```python
from build123d import *

# Parameters (mm, degrees)
SKETCH1_R           = 7.5
BOSS_EXTRUDE1_DEPTH = 16
SKETCH2_R           = 8.5
BOSS_EXTRUDE2_DEPTH = 2
SKETCH3_R           = 7
BOSS_EXTRUDE3_DEPTH = 35
SKETCH4_R           = 4
CUT_EXTRUDE1_DEPTH  = 20.5
SKETCH6_W           = 3
SKETCH6_H           = 1.5
CUT_EXTRUDE2_DEPTH  = 20.5
CUT_EXTRUDE3_REACH  = 18
SKETCH7_R           = 1
SKETCH8_W           = 3
SKETCH8_H           = 3
CUT_EXTRUDE5_DEPTH  = 33


with BuildPart() as part:
    # Sketch1 → Boss-Extrude1 (new body)
    with BuildSketch(Plane(origin=(0, 0, 0), x_dir=(0, 0, -1), z_dir=(1, 0, 0))):
        Circle(SKETCH1_R)
    extrude(amount=BOSS_EXTRUDE1_DEPTH)

    # Sketch2 → Boss-Extrude2 (add)
    with BuildSketch(Plane(origin=(16, 0, 0), x_dir=(0, 0, -1), z_dir=(1, 0, 0))):
        Circle(SKETCH2_R)
    extrude(amount=BOSS_EXTRUDE2_DEPTH)

    # Sketch3 → Boss-Extrude3 (add)
    with BuildSketch(Plane(origin=(18, 0, 0), x_dir=(0, 0, -1), z_dir=(1, 0, 0))):
        Circle(SKETCH3_R)
    extrude(amount=BOSS_EXTRUDE3_DEPTH)

    # Sketch4 → Cut-Extrude1 (cut)
    with BuildSketch(Plane.ZY):
        Circle(SKETCH4_R)
    extrude(amount=-CUT_EXTRUDE1_DEPTH, mode=Mode.SUBTRACT)

    # Sketch6 → Cut-Extrude2 (cut)
    with BuildSketch(Plane.ZY):
        with Locations((0, 4)):
            Rectangle(SKETCH6_W, SKETCH6_H)
    extrude(amount=-CUT_EXTRUDE2_DEPTH, mode=Mode.SUBTRACT)

    # Sketch7 → Cut-Extrude3 (cut, up to next)
    with BuildSketch(Plane(origin=(0, 7.5, 0), x_dir=(1, 0, 0), z_dir=(0, 1, 0)), mode=Mode.PRIVATE) as cut_extrude3_sk1:
        with Locations((9.6, 0)):
            Circle(SKETCH7_R)
    cut_extrude3_tool1 = extrude(cut_extrude3_sk1.sketch, amount=-CUT_EXTRUDE3_REACH, mode=Mode.PRIVATE) & part.part
    add(cut_extrude3_tool1.solids().sort_by_distance((9.6, 7.5, 0))[0], mode=Mode.SUBTRACT)

    # Sketch8 → Cut-Extrude5 (cut)
    with BuildSketch(Plane(origin=(53, 0, 0), x_dir=(0, 0, -1), z_dir=(1, 0, 0))):
        with Locations((0, -7)):
            Rectangle(SKETCH8_W, SKETCH8_H)
    extrude(amount=-CUT_EXTRUDE5_DEPTH, mode=Mode.SUBTRACT)


solid = part.part
```
CAD build for the part. Positions are in the model's coordinates, mm. A direction names the side the tool comes from. Give positions to 0.01 mm unless a question says otherwise; leave off trailing zeros. Write each loop counter-clockwise with the first axis right and the second up, starting at its lowest first coordinate (ties: lowest second). Pieces come first, ordered by that corner, then holes. Notation, with made-up numbers: (12, -11.5) -> (19, -11.5) arc R20 ccw to (19, 23.5) -> close; hole circle Ø6 at (56, 31). An arc over 180 degrees is marked (long way). Write each question's results on one line, items separated by ' | '.
1. Cut at C-C, the plane x = 12. Write the cut outline in (y, z).
Geometry check:
outline: circle Ø15 at (0, 0); hole (3.71, -1.5) -> (4.75, -1.5) -> (4.75, 1.5) -> (3.71, 1.5) arc R4 ccw (long way) to start
2. Drop flat-ended pins along their axis: P1, Ø0.7, axis at x = 39, y = -6, coming from the -Z side; P2, Ø6.5, axis at y = -1, z = -1, coming from the -X side; P3, Ø4, axis at x = 6.5, y = -2, coming from the -Z side; P4, Ø4, axis at x = 25, y = 4, coming from the -Z side. Give the stop position or say it passes through.
Geometry check:
P1: z = -4.13 | P2: x = 0 | P3: z = -7.5 | P4: z = -6.71
3. Cut at A-A, the plane z = 0. Write the cut outline in (x, y), then the cut area to 3 significant figures.
Geometry check:
outline: (0, -7.5) -> (16, -7.5) -> (16, -8.5) -> (18, -8.5) -> (18, -7) -> (20, -7) -> (20, -5.5) -> (53, -5.5) -> (53, 7) -> (18, 7) -> (18, 8.5) -> (16, 8.5) -> (16, 7.5) -> (10.6, 7.5) -> (10.6, 4.75) -> (20.5, 4.75) -> (20.5, -4) -> (0, -4) -> close; (0, 4.75) -> (8.6, 4.75) -> (8.6, 7.5) -> (0, 7.5) -> close | area: 530 mm²
4. Which spindle directions (+Z, -Z, +X, -X, +Y, -Y) get a long thin tool onto all of the face, cutting with end or side? Do faces 1 (the flat face through (53, 0, 0)), 2 (the flat face through (37, -6, 1.5)), 3 (the cylindrical face through (10.524, 6.144, 0.383)), 4 (the cylindrical face through (35.255, -2.681, -6.466)), 5 (the flat face through (16, -8, 0)). Say none if no direction does.
Geometry check:
face 1: +Z, -Z, +X, +Y, -Y | face 2: +X, -Y | face 3: +Y | face 4: +X | face 5: -X
5. Wall check: probe 1 along Y at (x, z) = (5.25, 0); probe 2 along Y at (x, z) = (19.5, 0.25); probe 3 along X at (y, z) = (-2, -0.25). Give the ranges that are in metal, low to high. Write a range as [from, to].
Geometry check:
probe 1: [-7.5, -4], [4.75, 7.5] | probe 2: [-7, -3.99], [4.75, 7] | probe 3: [20.5, 53]
6. Cut at B-B, the plane y = 0. Write the cut outline in (x, z).
Geometry check:
outline: (0, -7.5) -> (16, -7.5) -> (16, -8.5) -> (18, -8.5) -> (18, -7) -> (53, -7) -> (53, 7) -> (18, 7) -> (18, 8.5) -> (16, 8.5) -> (16, 7.5) -> (0, 7.5) -> (0, 4) -> (20.5, 4) -> (20.5, -4) -> (0, -4) -> close
7. Two-plate mould, pull along Y, no slides. Class faces 6 (the flat face through (20, -6, 0)), 7 (the cylindrical face through (7.89, -7.32, 1.63)), 8 (the flat face through (10, 4, -1.5)): pulls with the +Y half, pulls with the -Y half, needs draft (parallel to the pull), parting line crosses it, or undercut.
Geometry check:
face 6: needs draft | face 7: parting line crosses it | face 8: undercut
8. Cut at D-D, the plane z = 2.25. Write the cut outline in (x, y), then the cut area to 3 significant figures.
Geometry check:
outline: (0, -7.15) -> (16, -7.15) -> (16, -8.2) -> (18, -8.2) -> (18, -6.63) -> (53, -6.63) -> (53, 6.63) -> (18, 6.63) -> (18, 8.2) -> (16, 8.2) -> (16, 7.15) -> (0, 7.15) -> (0, 3.31) -> (20.5, 3.31) -> (20.5, -3.31) -> (0, -3.31) -> close | area: 590 mm²
